from build123d import *

# Parameters (mm, degrees)
F0_W      = 101.6
F0_H      = 101.6
F1_DEPTH  = 31.75
F2_R      = 9.525
F3_T      = -6.35
F8_DEPTH  = 6.35
F9_DEPTH  = 6.35
F10_DEPTH = 6.35
F11_DEPTH = 6.35


# Not quite as in the source:
# - a feature names something its author has since deleted; it is built from what else it names


with BuildPart() as f1:
    # F0 (on Top) → F1 (new body)
    with BuildSketch(Plane.XY):
        with Locations((50.8, -50.8)):
            Rectangle(F0_W, F0_H)
    extrude(amount=F1_DEPTH)

    # F2
    f2_edges = [f1.edges().sort_by_distance(p)[0] for p in [
        (0, -101.6, 15.875),
        (0, 0, 15.875),
        (101.6, 0, 15.875),
        (101.6, -101.6, 15.875),
    ]]
    fillet(f2_edges, radius=F2_R)

    # F3
    f3_openings = [f1.faces().sort_by_distance(p)[0] for p in [
        (50.8, -50.8, 0),
        (50.8, -50.8, 31.75),
    ]]
    offset(amount=F3_T, openings=f3_openings)

    # F6 (on face) → F8 (cut, through all)
    with BuildSketch(Plane(origin=(0, 0, 0), x_dir=(-1, 0, 0), z_dir=(0, 1, 0))):
        with BuildLine():
            Line((-50.8, 4.7625), (-90.4875, 4.7625))
            ThreePointArc((-90.4875, 4.7625), (-91.2928481737, 4.6939131403), (-92.075, 4.4901280605))
            Line((-92.075, 4.4901280605), (-92.075, 0))
            Line((-92.075, 0), (-9.525, 0))
            Line((-9.525, 0), (-9.525, 4.4901280605))
            ThreePointArc((-9.525, 4.4901280605), (-10.3071518263, 4.6939131403), (-11.1125, 4.7625))
            Line((-11.1125, 4.7625), (-50.8, 4.7625))
        make_face()
    extrude(amount=-F8_DEPTH, mode=Mode.SUBTRACT)

    # F7 (on face) → F9 (cut, through all)
    with BuildSketch(Plane.YZ.offset(101.6)):
        with BuildLine():
            Line((-50.8, 4.7625), (-90.4875, 4.7625))
            ThreePointArc((-90.4875, 4.7625), (-91.2928481737, 4.6939131403), (-92.075, 4.4901280605))
            Line((-92.075, 4.4901280605), (-92.075, 0))
            Line((-92.075, 0), (-9.525, 0))
            Line((-9.525, 0), (-9.525, 4.4901280605))
            ThreePointArc((-9.525, 4.4901280605), (-10.3071518263, 4.6939131403), (-11.1125, 4.7625))
            Line((-11.1125, 4.7625), (-50.8, 4.7625))
        make_face()
    extrude(amount=-F9_DEPTH, mode=Mode.SUBTRACT)

    # F4 (on face) → F10 (cut, through all)
    with BuildSketch(Plane.XZ.offset(101.6)):
        with BuildLine():
            Line((50.8, 4.7625), (17.4625, 4.7625))
            ThreePointArc((17.4625, 4.7625), (14.0949039546, 3.3675960454), (12.7, 0))
            Line((12.7, 0), (88.9, 0))
            ThreePointArc((88.9, 0), (87.5050960454, 3.3675960454), (84.1375, 4.7625))
            Line((84.1375, 4.7625), (50.8, 4.7625))
        make_face()
    extrude(amount=-F10_DEPTH, mode=Mode.SUBTRACT)

    # F5 (on face) → F11 (cut, through all)
    with BuildSketch(Plane(origin=(0, 0, 0), x_dir=(0, -1, 0), z_dir=(-1, 0, 0))):
        with BuildLine():
            Line((50.8, 4.7625), (23.8125, 4.7625))
            ThreePointArc((23.8125, 4.7625), (20.4449039546, 3.3675960454), (19.05, 0))
            Line((19.05, 0), (82.55, 0))
            ThreePointArc((82.55, 0), (81.1550960454, 3.3675960454), (77.7875, 4.7625))
            Line((77.7875, 4.7625), (50.8, 4.7625))
        make_face()
    extrude(amount=-F11_DEPTH, mode=Mode.SUBTRACT)


solid = f1.part
Model file for the job. Use its own axes, mm. A direction names the side the tool comes from. Give positions to 0.01 mm unless a question says otherwise; leave off trailing zeros. Loops run counter-clockwise (first coordinate to the right, second up) from the corner with the lowest first, then second, coordinate; pieces in that order, holes last.
1) Wall check: line 1 (X direction, y = -67, z = 24.5); line 2 (Y direction, x = 65.5, z = 6); line 3 (X direction, y = -5, z = 25.5). Give the ranges that are in metal, low to high.
2) Saw through at B-B (z = 24.5). Write the cut outline in (x, y) (3 decimals), plus the area to 3 significant figures.
3) Tool access for faces 1 (the cylindrical face through (94.3, -94.34, 16.1)), 2 (the flat face through (3, -51, 4.762)), 3 (the flat face through (51, -98, 4.762)): list every direction of +Z, -Z, +X, -X, +Y, -Y with a clear straight run to the whole face (end or side of a thin tool).
4) Flat gauge pins, fed straight in: pin 1 Ø3.5 at (y, z) = (-4, 3) entering from -X; pin 2 Ø2 at (x, z) = (97.5, 1.5) entering from +Y; pin 3 Ø5 at (y, z) = (-2, 1.5) entering from +X. Where does each tip first touch, or does it go through?
5) Pull direction Y, two halves, no side cores. Call faces 4 (the flat face through (101.6, -51, 18)), 5 (the flat face through (50, 0, 18)), 6 (the cylindrical face through (94, -7, 16)): +Y half, -Y half, draft (parallel to the pull), parting line (faces both ways), or undercut.
6) Saw through at C-C (y = -73). Write the cut outline in (x, z).
7) Saw through at A-A (x = 64). Write the cut outline in (y, z), plus the area to 3 significant figures.
Answer block:
1. line 1: x = 0 to 6.35, 95.25 to 101.6
1. line 2: y = -101.6 to -95.25, -6.35 to 0
1. line 3: x = 1.14 to 100.46
2. outline: (0, -92.075) arc R9.525 ccw to (9.525, -101.6) - (92.075, -101.6) arc R9.525 ccw to (101.6, -92.075) - (101.6, -9.525) arc R9.525 ccw to (92.075, 0) - (9.525, 0) arc R9.525 ccw to (0, -9.525) - close; hole (6.35, -92.075) arc R3.175 ccw to (9.525, -95.25) - (92.075, -95.25) arc R3.175 ccw to (95.25, -92.075) - (95.25, -9.525) arc R3.175 ccw to (92.075, -6.35) - (9.525, -6.35) arc R3.175 ccw to (6.35, -9.525) - close
2. area: 2,350 mm2
3. face 1: +Z, -Z
3. face 2: -Z, +X, -X
3. face 3: -Z, +Y, -Y
4. pin 1: stops at x = 0.78
4. pin 2: stops at y = -1.09
4. pin 3: stops at x = 100.17
5. face 4: draft
5. face 5: +Y half
5. face 6: undercut
6. outline: (0, 4.76) - (6.35, 4.76) - (6.35, 31.75) - (0, 31.75) - close; (95.25, 4.76) - (101.6, 4.76) - (101.6, 31.75) - (95.25, 31.75) - close
7. outline: (-101.6, 4.76) - (-95.25, 4.76) - (-95.25, 31.75) - (-101.6, 31.75) - close; (-6.35, 4.76) - (0, 4.76) - (0, 31.75) - (-6.35, 31.75) - close
7. area: 343 mm2
